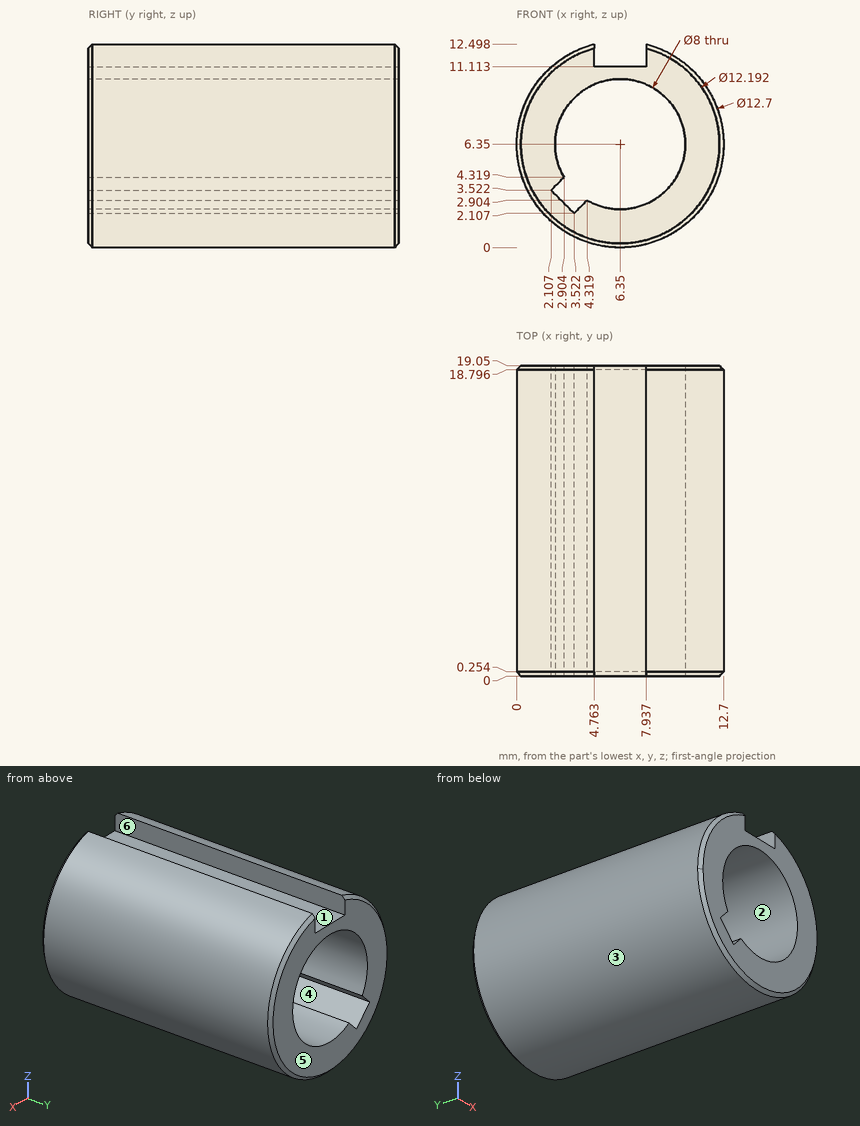
For this review, use the dimensioned drawing (mm, ordinates from the lowest corner) and the shaded views. A direction names the side the tool comes from. Round coordinates to 2 decimals unless told otherwise and drop trailing zeros. Answer as CSV lines item,"result".
1. Draft analysis for pull direction X (two halves, no side actions). For the marked faces 3, 4, 5 and 6, state which applies: pulls with the +X half, pulls with the -X half, needs draft (parallel to the pull), parting line crosses it, or undercut.
Outcome:
face 3,"parting line crosses it"
face 4,"undercut"
face 5,"needs draft"
face 6,"undercut"
2. For the marked faces 1 and 2, list the 3-axis set-ups (+Z, -Z, +X, -X, +Y, -Y) from which the entire face can be reached by the end or side of a thin tool; tool diameter is ignored.
Outcome:
face 1,"+Z, +Y, -Y"
face 2,"+Y, -Y"
3. To check wall thickness, follow L1, parallel to Z at x = 6.35, y = 5.5; L2, parallel to X at y = 6.75, z = 6.35; L3, parallel to X at y = 1, z = 4.5 (1 decimal). State the ranges of each line that lie inside material, in increasing order. Write a range as [from, to].
Outcome:
L1,"z = [0, 2.35], [10.35, 11.11]"
L2,"x = [0, 2.35], [10.35, 12.7]"
L3,"x = [0.3, 2.8], [9.9, 12.4]"
4. Insertion check: pin 1 Ø1.6 at (x, y) = (7, 12) entering from +Z; pin 2 Ø5 at (x, y) = (3.5, 3.5) entering from +Z; pin 3 Ø2 at (y, z) = (15.5, 10.5) entering from -X (1 decimal). Each pin has a flat end and moves straight along its axis. Give the tip position at first contact, or say it passes through.
Outcome:
pin 1,"stops at z = 11.11"
pin 2,"stops at z = 12.5"
pin 3,"stops at x = 0.8"
